The figure shows three views and two pictorial views of one solid part (mm, origin at its lowest corner). Answer the questions. Round coordinates to 2 decimals unless told otherwise and drop trailing zeros. Write each loop counter-clockwise with the first axis right and the second up, starting at its lowest first coordinate (ties: lowest second). Pieces come first, ordered by that corner, then holes. Notation, with made-up numbers: M 73,14.5 L 126,14.5 A20 ccw 126,34.5 Z; hole C -18,52 d10. An arc over 180 degrees is marked long. One line per item, written item: value. Start each with the question number.
Q1. The mould has two halves that part along Y. Classify the marked faces 1, 2, 3 and 4: released by +Y, released by -Y, zero draft, split by the parting line, or undercut.
Q2. Find section A-A (x = 5.25). Write down the section's boundary in (y, z) (1 decimal).
Q3. Given pin 1 Ø6 at (x, y) = (7, 5.5) entering from +Z, flat-ended and moving along its own axis, determine where the tip first touches the part or whether it passes through.
Q4. Find section C-C (z = 2). Write down the section's boundary in (x, y) (1 decimal).
Q5. Consider probe 1 along Y at (x, z) = (3.25, 1.65) (1 decimal); probe 2 along X at (y, z) = (8.25, 1.3) (1 decimal); probe 3 along X at (y, z) = (5.75, 0.2). Determine where each line is inside the solid, lowest interval first.
Q6. Find section B-B (y = 9). Write down the section's boundary in (x, z) (1 decimal).
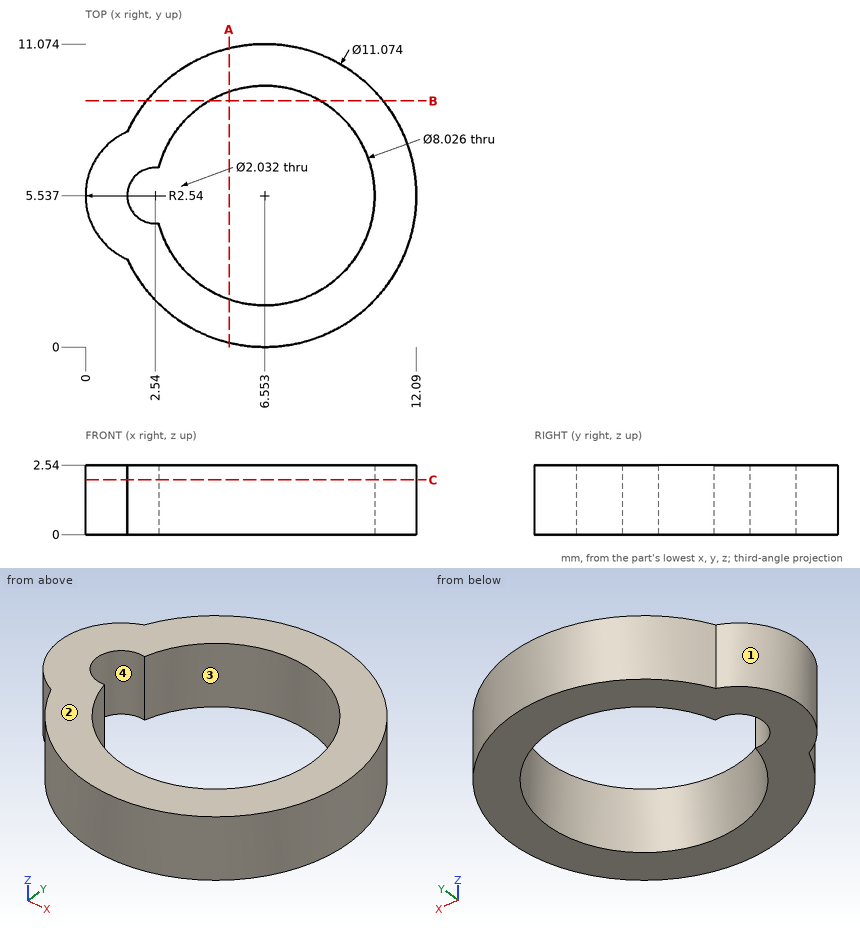
The answers:
1. face 1: split by the parting line
1. face 2: zero draft
1. face 3: undercut
1. face 4: undercut
2. outline: M 0.2,0 L 1.7,0 L 1.7,2.5 L 0.2,2.5 Z; M 9.3,0 L 10.9,0 L 10.9,2.5 L 9.3,2.5 Z
3. pin 1: through
4. outline: M 1.5,3.2 A5.5 ccw long 1.5,7.9 A2.5 ccw Z; hole M 2.7,4.5 A4 ccw long 2.7,6.5 A1 ccw long Z
5. probe 1: 1.1 to 3.3, 7.8 to 10
5. probe 2: 1.7 to 3.6, 9.5 to 11.4
5. probe 3: 0.01 to 1.55, 10.56 to 12.09
6. outline: M 2.2,0 L 4.5,0 L 4.5,2.5 L 2.2,2.5 Z; M 8.6,0 L 10.9,0 L 10.9,2.5 L 8.6,2.5 Z
